Input: part model. Units: mm. Frame: model coordinates. Face numbers are marked on the shaded views. Give positions to 0.01 mm unless a question says otherwise; leave off trailing zeros. Write each loop counter-clockwise with the first axis right and the second up, starting at its lowest first coordinate (ties: lowest second). Pieces come first, ordered by that corner, then holes. Notation, with made-up numbers: M 10.25,-9 L 41.25,-9 A33 ccw 41.25,19 Z; hole C 24,-1.75 d10. An arc over 180 degrees is marked long. Use CSV: the item, a comma, the result in double quotes. Start each with the question number.
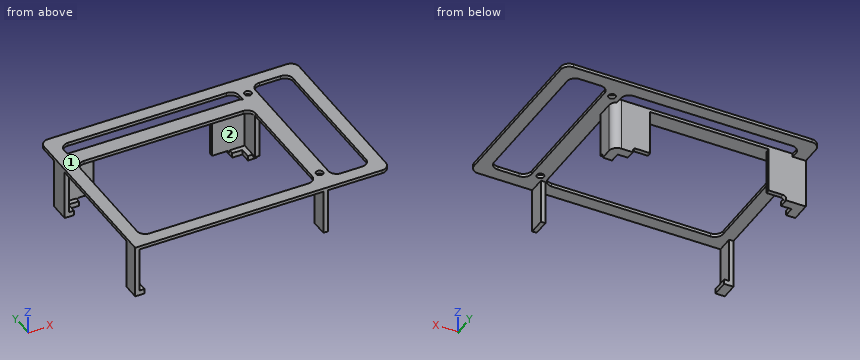
from build123d import *

# Parameters (mm, degrees)
SKETCH1_W             = 156.3
SKETCH1_H             = 110
SKETCH1_W_2           = 107.3
SKETCH1_H_2           = 75.3
SKETCH1_H_3           = 8.7
SKETCH1_W_3           = 23
SKETCH1_H_4           = 94
BOSS_EXTRUDE1_DEPTH   = 2
F_6_CLEARANCE_HOLE1_D = 4.3053
SKETCH6_W             = 2.7
SKETCH6_H             = 10
BOSS_EXTRUDE2_DEPTH   = 27.6
SKETCH7_W             = 5.7
SKETCH7_H             = 10
BOSS_EXTRUDE3_DEPTH   = 3
FILLET3_R             = 5
FILLET4_R             = 2
FILLET5_R             = 5


with BuildPart() as part:
    # Sketch1 → Boss-Extrude1 (new body)
    with BuildSketch(Plane.XY):
        with Locations((78.15, 55)):
            Rectangle(SKETCH1_W, SKETCH1_H)
        with Locations((61.65, 45.65)):
            Rectangle(SKETCH1_W_2, SKETCH1_H_2, mode=Mode.SUBTRACT)
        with Locations((61.65, 97.65)):
            Rectangle(SKETCH1_W_2, SKETCH1_H_3, mode=Mode.SUBTRACT)
        with Locations((136.8, 55)):
            Rectangle(SKETCH1_W_3, SKETCH1_H_4, mode=Mode.SUBTRACT)
    extrude(amount=BOSS_EXTRUDE1_DEPTH)

    # #6 Clearance Hole1 (through all)
    with Locations(Plane(origin=(0, 0, 0), x_dir=(-1, 0, 0), z_dir=(0, 0, -1))):
        with Locations((-120.3, 13.725), (-120.3, 96.275)):
            Hole(F_6_CLEARANCE_HOLE1_D / 2)

    # Sketch6 → Boss-Extrude2 (add)
    with BuildSketch(Plane(origin=(0, 0, 0), x_dir=(-1, 0, 0), z_dir=(0, 0, -1))):
        with Locations((-1.35, 5)):
            Rectangle(SKETCH6_W, SKETCH6_H)
        with Locations((-116.65, 5)):
            Rectangle(SKETCH6_W, SKETCH6_H)
        Polygon((0, 81.3), (0, 93.3), (-22.7, 93.3), (-22.7, 90.6), (-2.7, 90.6), (-2.7, 81.3), align=None)
        Polygon((-95.3, 93.3), (-118, 93.3), (-118, 78.6), (-115.3, 78.6), (-115.3, 90.6), (-95.3, 90.6), align=None)
    extrude(amount=BOSS_EXTRUDE2_DEPTH)

    # Sketch7 → Boss-Extrude3 (add)
    with BuildSketch(Plane(origin=(0, 0, -27.6), x_dir=(-1, 0, 0), z_dir=(0, 0, -1))):
        Polygon((0, 93.3), (0, 81.3), (-5.7, 81.3), (-5.7, 87.6), (-12, 87.6), (-12, 93.3), align=None)
        with Locations((-2.85, 5)):
            Rectangle(SKETCH7_W, SKETCH7_H)
        Polygon((-118, 93.3), (-118, 81.3), (-112.3, 81.3), (-112.3, 87.6), (-106, 87.6), (-106, 93.3), align=None)
    extrude(amount=BOSS_EXTRUDE3_DEPTH)

    # Fillet3
    fillet3_edges = [part.edges().sort_by_distance(p)[0] for p in [
        (118, 93.3, -15.3),
    ]]
    fillet(fillet3_edges, radius=FILLET3_R)

    # Fillet4
    fillet4_edges = [part.edges().sort_by_distance(p)[0] for p in [
        (12, 91.95, -27.6),
        (106, 91.95, -27.6),
        (116.65, 81.3, -27.6),
    ]]
    fillet(fillet4_edges, radius=FILLET4_R)

    # Fillet5
    # the kernel refuses this fillet: 5 mm, written as the material it adds along each edge
    with BuildSketch(Plane(origin=(8, 83.3, 0), x_dir=(1, 0, 0), z_dir=(0, 0, 1)), Plane(origin=(115.3, 83.3, 0), x_dir=(0, -1, 0), z_dir=(0, 0, 1)), Plane(origin=(148.3, 102, 0), x_dir=(0, -1, 0), z_dir=(0, 0, 1)), Plane(origin=(148.3, 8, 0), x_dir=(-1, 0, 0), z_dir=(0, 0, 1)), Plane(origin=(8, 102, 0), x_dir=(1, 0, 0), z_dir=(0, 0, 1)), Plane(origin=(115.3, 102, 0), x_dir=(0, -1, 0), z_dir=(0, 0, 1))) as fillet5_piece_1:
        with BuildLine():
            CenterArc((FILLET5_R, -FILLET5_R), FILLET5_R, 90, 90)
            Line((0, -FILLET5_R), (0, 0))
            Line((0, 0), (FILLET5_R, 0))
        make_face()
    extrude(amount=2)
    with BuildSketch(Plane(origin=(8, 8, 0), x_dir=(1, 0, 0), z_dir=(0, 0, 1)), Plane(origin=(115.3, 8, 0), x_dir=(0, 1, 0), z_dir=(0, 0, 1)), Plane(origin=(125.3, 102, 0), x_dir=(0, -1, 0), z_dir=(0, 0, 1)), Plane(origin=(125.3, 8, 0), x_dir=(1, 0, 0), z_dir=(0, 0, 1))) as fillet5_piece_2:
        with BuildLine():
            CenterArc((FILLET5_R, FILLET5_R), FILLET5_R, 180, 90)
            Line((0, FILLET5_R), (0, 0))
            Line((0, 0), (FILLET5_R, 0))
        make_face()
    extrude(amount=2)
    # the kernel refuses this fillet: 5 mm, written as the material it takes off along each edge
    with BuildSketch(Plane(origin=(0, 110, -12.5), x_dir=(1, 0, 0), z_dir=(0, 0, 1))) as fillet5_2_piece_1:
        with BuildLine():
            CenterArc((FILLET5_R, -FILLET5_R), FILLET5_R, 90, 90)
            Line((0, -FILLET5_R), (0, 0))
            Line((0, 0), (FILLET5_R, 0))
        make_face()
    extrude(amount=27, mode=Mode.SUBTRACT)
    with BuildSketch(Plane(origin=(156.3, 110, -12.5), x_dir=(-1, 0, 0), z_dir=(0, 0, 1)), Plane(origin=(156.3, 0, -12.5), x_dir=(0, 1, 0), z_dir=(0, 0, 1))) as fillet5_2_piece_2:
        with BuildLine():
            CenterArc((FILLET5_R, FILLET5_R), FILLET5_R, 180, 90)
            Line((0, FILLET5_R), (0, 0))
            Line((0, 0), (FILLET5_R, 0))
        make_face()
    extrude(amount=27, mode=Mode.SUBTRACT)


solid = part.part
Q1. Section A-A, the plane y = 34.5. Return the cut outline in (x, z), and give its area (3 significant figures).
Q2. Pull-direction query (X, two-part tool) for the marked faces 1 and 2; classes: released by +X, released by -X, zero draft, split by the parting line, or undercut.
Q3. Section C-C, the plane z = -10.5. Return the cut outline in (x, y), and give its area (3 significant figures).
Q4. Section B-B, the plane x = 120.3. Return the cut outline in (y, z).
Q5. Section D-D, the plane x = 139.5. Return the cut outline in (y, z), and give its area (3 significant figures).
Q6. First-contact query: pin 1 Ø6.5 at (x, z) = (4, -10.5) entering from -Y; pin 2 Ø1.5 at (y, z) = (7.5, -29) entering from +X; pin 3 Ø1.4 at (x, y) = (17.5, 91.5) entering from -Z; pin 4 Ø3.5 at (x, y) = (120.3, 13.725) entering from +Z. Flat tips, straight axial feed; report the tip coordinate or a pass-through.
Q7. Material intervals for L1, parallel to Y at x = 120, z = 1; L2, parallel to Y at x = 87, z = 1; L3, parallel to Y at x = 112, z = -19, sorted ascending. Write a range as [from, to].
Check result:
1,outline,"M 0,0 L 8,0 L 8,2 L 0,2 Z; M 115.3,0 L 125.3,0 L 125.3,2 L 115.3,2 Z; M 148.3,0 L 156.3,0 L 156.3,2 L 148.3,2 Z"
1,area,"52.0 mm²"
2,face 1,"zero draft"
2,face 2,"undercut"
3,outline,"M 0,0 L 2.7,0 L 2.7,10 L 0,10 Z; M 0,81.3 L 2.7,81.3 L 2.7,90.6 L 22.7,90.6 L 22.7,93.3 L 0,93.3 Z; M 95.3,90.6 L 115.3,90.6 L 115.3,78.6 L 118,78.6 L 118,88.3 A5 ccw 113,93.3 L 95.3,93.3 Z; M 115.3,0 L 118,0 L 118,10 L 115.3,10 Z"
3,area,"229 mm²"
4,outline,"M 0,0 L 11.57,0 L 11.57,2 L 0,2 Z; M 15.88,0 L 94.12,0 L 94.12,2 L 15.88,2 Z; M 98.43,0 L 110,0 L 110,2 L 98.43,2 Z"
5,outline,"M 0,0 L 8,0 L 8,2 L 0,2 Z; M 102,0 L 110,0 L 110,2 L 102,2 Z"
5,area,"32.0 mm²"
6,pin 1,"stops at y = 0"
6,pin 2,"stops at x = 5.7"
6,pin 3,"stops at z = -27.6"
6,pin 4,"passes through"
7,L1,"y = [0, 11.59], [15.86, 94.14], [98.41, 110]"
7,L2,"y = [0, 8], [83.3, 93.3], [102, 110]"
7,L3,"y = [90.6, 93.3]"
